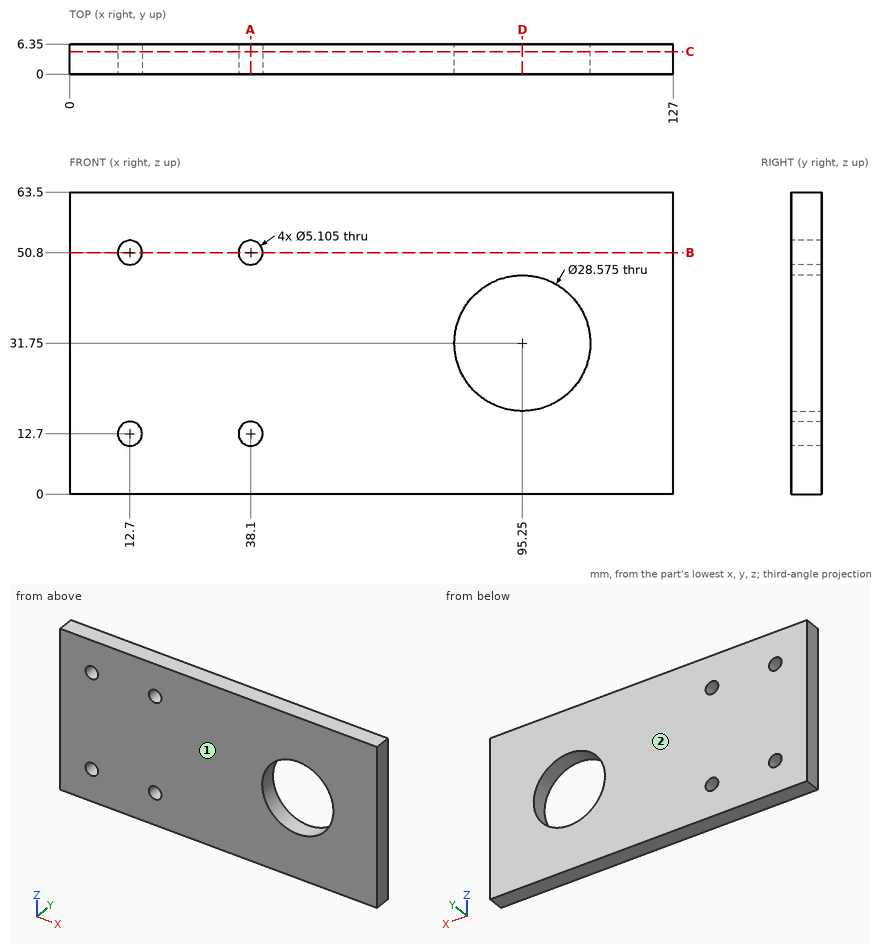
Part print with two shaded views. Sizes in mm from the minimum x, y, z corner. Coordinates: 2 decimals unless noted, no trailing zeros. Write each loop counter-clockwise with the first axis right and the second up, starting at its lowest first coordinate (ties: lowest second). Pieces come first, ordered by that corner, then holes.
1. Drill centre lines: probe 1 along Z at (x, y) = (12.7, 5.25); probe 2 along X at (y, z) = (4.75, 50.8); probe 3 along X at (y, z) = (1.75, 13.5) (1 decimal). Where is each one in solid material? Low to high.
Answer block:
probe 1: z = 0 to 10.15, 15.25 to 48.25, 53.35 to 63.5
probe 2: x = 0 to 10.15, 15.25 to 35.55, 40.65 to 127
probe 3: x = 0 to 10.3, 15.1 to 35.7, 40.5 to 127
2. Pull direction Y, two halves, no side cores. Call the marked faces 1 and 2: released by +Y, released by -Y, zero draft, split by the parting line, or undercut.
Answer block:
face 1: released by -Y
face 2: released by +Y
3. Band-saw the part on A-A, the plane x = 38.1. Give the cut face in (y, z).
Answer block:
outline: (0, 0) - (6.35, 0) - (6.35, 10.15) - (0, 10.15) - close; (0, 15.25) - (6.35, 15.25) - (6.35, 48.25) - (0, 48.25) - close; (0, 53.35) - (6.35, 53.35) - (6.35, 63.5) - (0, 63.5) - close
4. Band-saw the part on D-D, the plane x = 95.25. Give the cut face in (y, z).
Answer block:
outline: (0, 0) - (6.35, 0) - (6.35, 17.46) - (0, 17.46) - close; (0, 46.04) - (6.35, 46.04) - (6.35, 63.5) - (0, 63.5) - close
5. Band-saw the part on B-B, the plane z = 50.8. Give the cut face in (x, y).
Answer block:
outline: (0, 0) - (10.15, 0) - (10.15, 6.35) - (0, 6.35) - close; (15.25, 0) - (35.55, 0) - (35.55, 6.35) - (15.25, 6.35) - close; (40.65, 0) - (127, 0) - (127, 6.35) - (40.65, 6.35) - close
6. Band-saw the part on C-C, the plane y = 4.75. Give the number of separate pieces and of enclosed holes in the cut face, and give its area (3 significant figures).
Answer block:
separate pieces: 1
enclosed holes: 5
area: 7,340 mm2
